Can you work these out from the drawing? Everything is in mm from the part's minimum corner. A direction names the side the tool comes from. Coordinates: 2 decimals unless noted, no trailing zeros. Write each loop counter-clockwise with the first axis right and the second up, starting at its lowest first coordinate (ties: lowest second). Pieces come first, ordered by that corner, then holes.
(1) Imagine slicing it at C-C, the plane y = 50.5. List the corners of the cut face in (x, z) for me.
(2) Imagine slicing it at D-D, the plane x = 60. List the corners of the cut face in (y, z) for me, plus the area to 3 significant figures.
(3) Please list where these lines run through material, in increasing order: probe 1 along Z at (x, y) = (45, 1); probe 2 along X at (y, z) = (1.15, 59); probe 3 along Y at (x, z) = (100, 5).
(4) Which directions (+Z, -Z, +X, -X, +Y, -Y) give clear straight access to the entire face, cutting with the end or side of a thin tool? Please do the marked faces 1, 2, 3 and 4.
(5) For pin 1 Ø10 at (x, z) = (112.5, 24.5) entering from +Y; pin 2 Ø2 at (y, z) = (0.5, 60.5) entering from -X; pin 3 Ø3 at (x, z) = (115, 59) entering from +Y; pin 4 Ø1.6 at (x, y) = (141.5, 1) entering from -Z, each with a flat end and sliding along its axis, tell me the tip position at first contact or that it passes through.
(6) Imagine slicing it at A-A, the plane x = 115. List the corners of the cut face in (y, z) for me.
(7) Thinking about a two-plate mould opening in X: for the marked faces 5, 6 and 7, which applies, released by +X, released by -X, zero draft, split by the parting line, or undercut?
(8) Imagine slicing it at B-B, the plane z = 4. List the corners of the cut face in (x, y) for me.
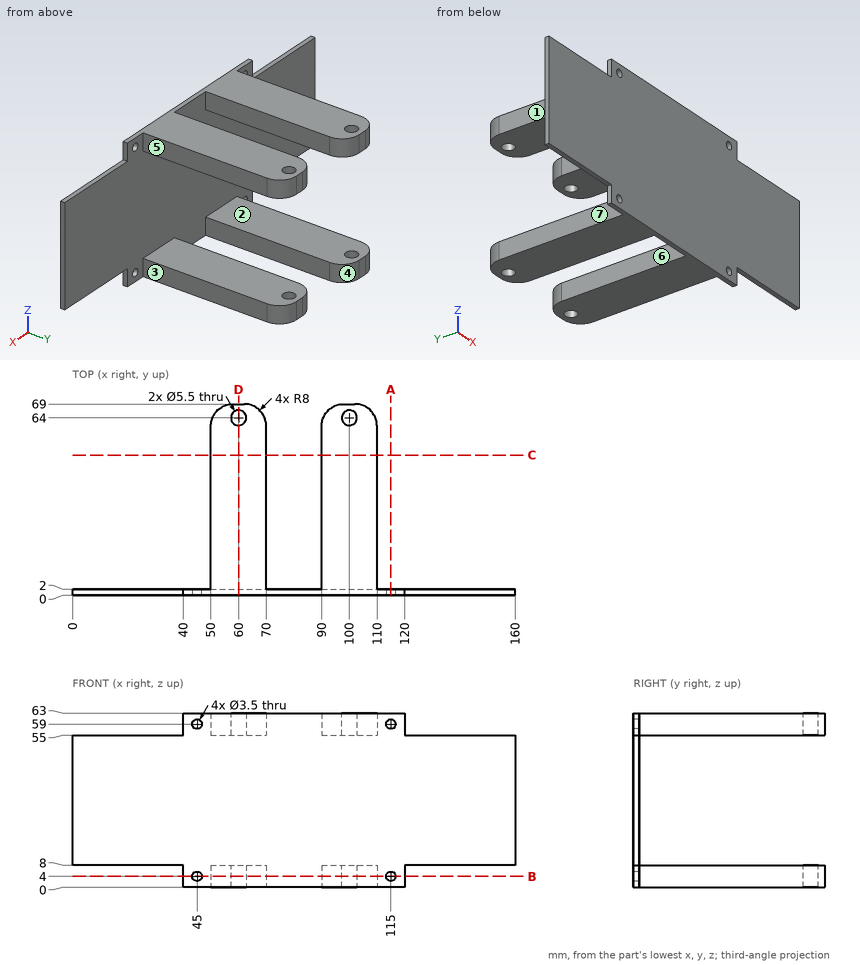
Recorded:
1. outline: (50, 0) - (70, 0) - (70, 8) - (50, 8) - close; (50, 55) - (70, 55) - (70, 63) - (50, 63) - close; (90, 0) - (110, 0) - (110, 8) - (90, 8) - close; (90, 55) - (110, 55) - (110, 63) - (90, 63) - close
2. outline: (0, 0) - (61.25, 0) - (61.25, 8) - (2, 8) - (2, 55) - (61.25, 55) - (61.25, 63) - (0, 63) - close; (66.75, 0) - (69, 0) - (69, 8) - (66.75, 8) - close; (66.75, 55) - (69, 55) - (69, 63) - (66.75, 63) - close
2. area: 1,110 mm2
3. probe 1: z = 0 to 2.25, 5.75 to 57.25, 60.75 to 63
3. probe 2: x = 40 to 43.25, 46.75 to 113.25, 116.75 to 120
3. probe 3: y = 0 to 61.25, 66.75 to 69
4. face 1: +Z, -Z, -X, +Y
4. face 2: +X, -X, +Y
4. face 3: +Z, -Z, +X, +Y
4. face 4: +Z, -Z, +Y
5. pin 1: stops at y = 2
5. pin 2: stops at x = 40
5. pin 3: passes through
5. pin 4: stops at z = 8
6. outline: (0, 0) - (2, 0) - (2, 2.25) - (0, 2.25) - close; (0, 5.75) - (2, 5.75) - (2, 57.25) - (0, 57.25) - close; (0, 60.75) - (2, 60.75) - (2, 63) - (0, 63) - close
7. face 5: released by +X
7. face 6: undercut
7. face 7: released by -X
8. outline: (40, 0) - (43.25, 0) - (43.25, 2) - (40, 2) - close; (46.75, 0) - (113.25, 0) - (113.25, 2) - (110, 2) - (110, 61) arc R8 ccw to (102, 69) - (98, 69) arc R8 ccw to (90, 61) - (90, 2) - (70, 2) - (70, 61) arc R8 ccw to (62, 69) - (58, 69) arc R8 ccw to (50, 61) - (50, 2) - (46.75, 2) - close; (116.75, 0) - (120, 0) - (120, 2) - (116.75, 2) - close; hole circle Ø5.5 at (60, 64); hole circle Ø5.5 at (100, 64)
